Read the model definition and answer for the solid it produces. Units are mm, in the model's axes. Face numbers are marked on the shaded views. A direction names the side the tool comes from. Coordinates: 2 decimals unless noted, no trailing zeros. Order: outer loops, then holes, each group sorted by start corner. A loop starts at its lowest first (then second) coordinate and runs counter-clockwise, first axis right, second up. Notation, with made-up numbers: (-38, 28.5) -> (20, 28.5) arc R28 ccw to (20, 55.5) -> close; hole circle Ø9 at (15, 15.5). An arc over 180 degrees is marked (long way). Answer in a Markdown table with one row per item.
from build123d import *

# Parameters (mm, degrees)
F0_W      = 51.7292671493
F0_H      = 12.7
F1_DEPTH  = 25.4
F3_DEPTH  = 12.7
F4_DEPTH  = 25.4
F5_W      = 25.4
F5_H      = 25.4
F6_DEPTH  = 19.05
F8_DEPTH  = 25.4
F9_R      = 6.35
F10_DEPTH = 25.4
F11_R     = 6.35
F12_DEPTH = 25.4
F13_R     = 6.35
F14_DEPTH = 25.4


with BuildPart() as f1:
    # F0 (on Front) → F1 (new body)
    with BuildSketch(Plane.XZ):
        with Locations((-25.8646335747, 6.35)):
            Rectangle(F0_W, F0_H)
    extrude(amount=F1_DEPTH)

    # F2 (on face) → F3 (join)
    with BuildSketch(Plane.XY.offset(12.7)):
        with BuildLine():
            ThreePointArc((-51.7292671493, 0), (-64.4292671493, -12.7), (-51.7292671493, -25.4))
            Line((-51.7292671493, -25.4), (-51.7292671493, 0))
        make_face()
        with BuildLine():
            Line((0, 0), (0, -25.4))
            ThreePointArc((0, -25.4), (12.7, -12.7), (0, 0))
        make_face()
    extrude(amount=-F3_DEPTH)

    # F0 (on Front) → F4 (join)
    with BuildSketch(Plane.XZ):
        with Locations((-25.8646335747, 6.35)):
            Rectangle(F0_W, F0_H)
    extrude(amount=F4_DEPTH)

    # F5 (on face) → F6 (join)
    with BuildSketch(Plane.XY.offset(12.7)):
        with Locations((-28.0921224833, -12.7)):
            Rectangle(F5_W, F5_H)
    extrude(amount=F6_DEPTH)

    # F7 (on face) → F8 (join)
    with BuildSketch(Plane.YZ.offset(-15.3921224833)):
        with BuildLine():
            Line((-25.4, 31.75), (0, 31.75))
            ThreePointArc((0, 31.75), (-12.7, 44.45), (-25.4, 31.75))
        make_face()
    extrude(amount=-F8_DEPTH)

    # F9 (on face) → F10 (cut)
    with BuildSketch(Plane.YZ.offset(-15.3921224833)):
        with Locations((-12.7, 31.75)):
            Circle(F9_R)
    extrude(amount=-F10_DEPTH, mode=Mode.SUBTRACT)

    # F11 (on face) → F12 (cut)
    with BuildSketch(Plane.XY.offset(12.7)):
        with Locations((0, -12.7)):
            Circle(F11_R)
    extrude(amount=-F12_DEPTH, mode=Mode.SUBTRACT)

    # F13 (on face) → F14 (cut)
    with BuildSketch(Plane.XY.offset(12.7)):
        with Locations((-51.7292671493, -12.7)):
            Circle(F13_R)
    extrude(amount=-F14_DEPTH, mode=Mode.SUBTRACT)


solid = f1.part
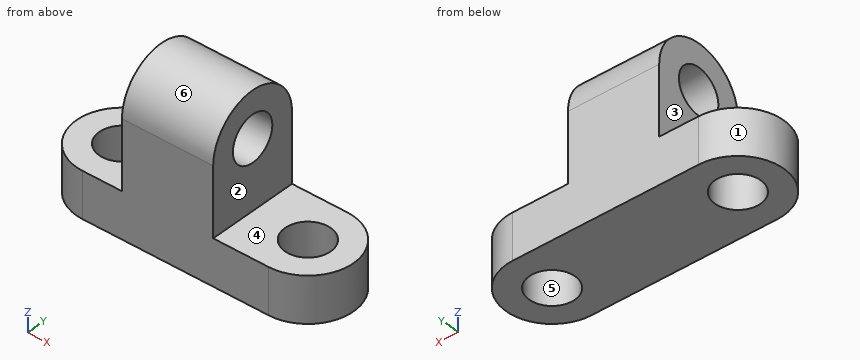
Q1. The part is cut by section D-D (z = 4). Write down the section's boundary in (x, y).
Outcome:
| item | result |
|---|---|
| outline | (-51.73, -25.4) -> (0, -25.4) arc R12.7 ccw to (0, 0) -> (-51.73, 0) arc R12.7 ccw to start; hole circle Ø12.7 at (-51.73, -12.7); hole circle Ø12.7 at (0, -12.7) |
Q2. The part is cut by section C-C (z = 34). Write down the section's boundary in (x, y), then the cut area to 3 significant figures.
Outcome:
| item | result |
|---|---|
| outline | (-40.79, -25.2) -> (-15.39, -25.2) -> (-15.39, -18.64) -> (-40.79, -18.64) -> close; (-40.79, -6.76) -> (-15.39, -6.76) -> (-15.39, -0.2) -> (-40.79, -0.2) -> close |
| area | 333 mm² |
Q3. For the marked faces 1, 2 and 3, determine the directions among +Z, -Z, +X, -X, +Y, -Y from which every point of the face is accessible in a straight line to the end or side of a thin tool.
Outcome:
| item | result |
|---|---|
| face 1 | +Z, -Z, -X |
| face 2 | +Z, +X, +Y, -Y |
| face 3 | +Z, -X, +Y, -Y |
Q4. The part is cut by section B-B (x = -18). Write down the section's boundary in (y, z).
Outcome:
| item | result |
|---|---|
| outline | (-25.4, 0) -> (0, 0) -> (0, 31.75) arc R12.7 ccw to (-25.4, 31.75) -> close; hole circle Ø12.7 at (-12.7, 31.75) |
Q5. For a pull along Y with two mould halves and no side action, classify the marked faces 4, 5 and 6 as pulls with the +Y half, pulls with the -Y half, needs draft (parallel to the pull), parting line crosses it, or undercut.
Outcome:
| item | result |
|---|---|
| face 4 | needs draft |
| face 5 | undercut |
| face 6 | parting line crosses it |
Q6. Consider line 1 (Z direction, x = -31.5, y = -12.7); line 2 (Y direction, x = -52, z = 8.5); line 3 (X direction, y = -15.25, z = 7). Determine where each line is inside the solid, lowest interval first.
Outcome:
| item | result |
|---|---|
| line 1 | 0 to 25.4, 38.1 to 44.45 |
| line 2 | -25.4 to -19.04, -6.36 to 0 |
| line 3 | -64.17 to -57.54, -45.91 to -5.82, 5.82 to 12.44 |
Q7. Given pin 1 (6 mm diameter, centred on y = -17, z = 19, fed in from +X); pin 2 (10 mm diameter, centred on x = -23, y = -22, fed in from +Z); pin 3 (5 mm diameter, centred on x = -17, y = -5, fed in from +Z), each flat-ended and moving along its own axis, determine where each tip first touches the part or whether it passes through.
Outcome:
| item | result |
|---|---|
| pin 1 | x = -15.39 |
| pin 2 | z = 43.7 |
| pin 3 | z = 43.34 |
Q8. The part is cut by section A-A (y = -12.7). Write down the section's boundary in (x, z).
Outcome:
| item | result |
|---|---|
| outline | (-64.43, 0) -> (-58.08, 0) -> (-58.08, 12.7) -> (-64.43, 12.7) -> close; (-45.38, 0) -> (-6.35, 0) -> (-6.35, 12.7) -> (-15.39, 12.7) -> (-15.39, 25.4) -> (-40.79, 25.4) -> (-40.79, 12.7) -> (-45.38, 12.7) -> close; (-40.79, 38.1) -> (-15.39, 38.1) -> (-15.39, 44.45) -> (-40.79, 44.45) -> close; (6.35, 0) -> (12.7, 0) -> (12.7, 12.7) -> (6.35, 12.7) -> close |
